Autodesk Inventor part; units mm, degrees
ref_plane "YZ Plane" through (0, 0, 0) normal (1, 0, 0) x (0, 1, 0)
ref_plane "XZ Plane" through (0, 0, 0) normal (0, 1, 0) x (-1, 0, 0)
ref_plane "XY Plane" through (0, 0, 0) normal (0, 0, 1) x (1, 0, 0)
sketch "Esquisse1" plane through (0, 0, 0) normal (0, 1, 0) x (-1, 0, 0)
  line L0 (0, 0) -> (0, 45)
  line L1 (0, 45) -> (45, 45)
  line L2 (0, 0) -> (128, -75.3746)
  line L3 (45, 45) -> (155, -30.3746)
  line L4 (155, -30.3746) -> (171.5194, -75.3746)
  line L5 (128, -75.3746) -> (137.66, -105.3746)
  line L6 (137.66, -105.3746) -> (177.0258, -90.3746)
  line L7 (171.5194, -75.3746) -> (183.1092, -79.0397)
  line L8 (183.1092, -79.0397) -> (186.1095, -86.9134)
  line L9 (186.1095, -86.9134) -> (177.0258, -90.3746)
  dimension "d0" = 45
  dimension "d1" = 45
  dimension "d13" = 128
  dimension "d14" = 110
  dimension "d15" = 30
  dimension "d16" = 45
extrude "Extrusion1" add sketch "Esquisse1" along normal blind 3
sketch "Esquisse2" plane through (0, 3, 0) normal (0, 1, 0) x (1, 0, 0)
  line L0 (-164.1382, 85.6541) -> (-143.0194, 93.7013)
  line L1 (-159.8297, 74.3472) -> (-138.7109, 82.3943)
  line L2 (-137.66, 105.3746) -> (-186.1095, 86.9134)
  line L3 (-138.7109, 82.3943) -> (-143.0194, 93.7013)
  line L4 (-159.8297, 74.3472) -> (-164.1382, 85.6541)
  point P0 (0, 0)
  dimension "d19" = 9
  dimension "d20" = 9
  dimension "d22" = 12.1
  dimension "d23" = 12.1
  dimension "d24" = 22.6
extrude "Extrusion2" cut sketch "Esquisse2" against normal blind 3
Design review of the part built by this model. Coordinates are the model's own, in mm. A direction names the side the tool comes from. Coordinates: 2 decimals unless noted, no trailing zeros. Order: outer loops, then holes, each group sorted by start corner. A loop starts at its lowest first (then second) coordinate and runs counter-clockwise, first axis right, second up. Notation, with made-up numbers: M -1.75,-0.75 L 4.25,-0.75 A25 cw 4.25,11.25 Z; hole C -7.5,28 d7. An arc over 180 degrees is marked long. Use a Markdown table: item, result.
(1) Add section B-B (z = -25). Give the boundary of the cut face in (x, y), then the cut area to 3 significant figures.
Worked answers:
| item | result |
|---|---|
| outline | M -147.16,0 L -42.45,0 L -42.45,3 L -147.16,3 Z |
| area | 314 mm2 |
(2) Draft analysis for pull direction X (two halves, no side actions). For faces 1 (the flat face through (-92, 0, -12)), 2 (the flat face through (-163.144, 1.479, -52.56)), 3 (the flat face through (-161.954, 1.521, -79.922)), state which applies: released by +X, released by -X, zero draft, split by the parting line, or undercut.
Worked answers:
| item | result |
|---|---|
| face 1 | zero draft |
| face 2 | released by -X |
| face 3 | undercut |
(3) Wall thickness on probe 1 along X at (y, z) = (1.85, -54); probe 2 along Z at (x, y) = (-100, 0.2); probe 3 along X at (y, z) = (2.5, -29): over which ranges is each line inside the solid? List them lowest first.
Worked answers:
| item | result |
|---|---|
| probe 1 | x = -163.67 to -91.7 |
| probe 2 | z = -58.89 to 7.31 |
| probe 3 | x = -152.99 to -49.25 |
(4) Add section C-C (x = -22.5). Give the boundary of the cut face in (y, z).
Worked answers:
| item | result |
|---|---|
| outline | M 0,-13.25 L 3,-13.25 L 3,45 L 0,45 Z |
(5) For faces 4 (the flat face through (-63.104, 1.479, -37.16)), 5 (the flat face through (-149.418, 1.521, -78.314)), list the 3-axis set-ups (+Z, -Z, +X, -X, +Y, -Y) from which the entire face can be reached by the end or side of a thin tool; tool diameter is ignored.
Worked answers:
| item | result |
|---|---|
| face 4 | -Z, +X, +Y, -Y |
| face 5 | +Y, -Y |
(6) Add section A-A (y = 1.95). Give the boundary of the cut face in (x, z), then the cut area to 3 significant figures.
Worked answers:
| item | result |
|---|---|
| outline | M -186.11,-86.91 L -177.03,-90.37 L -137.66,-105.37 L -128,-75.37 L 0,0 L 0,45 L -45,45 L -155,-30.37 L -171.52,-75.37 L -183.11,-79.04 Z; hole M -164.14,-85.65 L -143.02,-93.7 L -138.71,-82.39 L -159.83,-74.35 Z |
| area | 10,900 mm2 |
